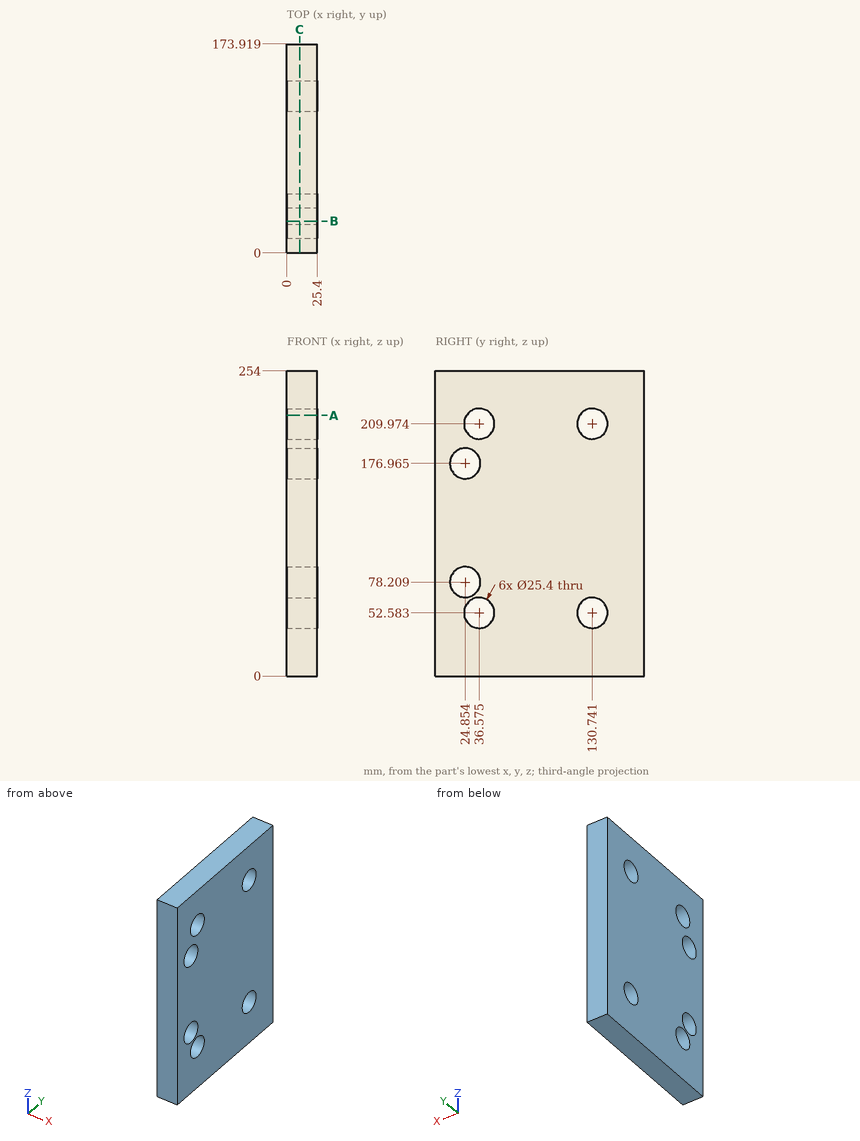
Drawing for the job (mm, zero at the part's lowest x, y, z). Round coordinates to 2 decimals unless told otherwise and drop trailing zeros. Write each loop counter-clockwise with the first axis right and the second up, starting at its lowest first coordinate (ties: lowest second). Pieces come first, ordered by that corner, then holes.
Item 1: Band-saw the part on B-B on y = 26.5. Give the number of separate pieces and of enclosed holes in the cut face, then the cut area to 3 significant figures.
Filled in:
separate pieces: 5
enclosed holes: 0
area: 4,390 mm2
Item 2: Band-saw the part on A-A on z = 217. Write the cut outline in (x, y) (1 decimal), then the cut area to 3 significant figures.
Filled in:
outline: (0, 0) - (25.4, 0) - (25.4, 26) - (0, 26) - close; (0, 47.2) - (25.4, 47.2) - (25.4, 120.2) - (0, 120.2) - close; (0, 141.3) - (25.4, 141.3) - (25.4, 173.9) - (0, 173.9) - close
area: 3,340 mm2
Item 3: Drill centre lines: L1, parallel to Y at x = 16.25, z = 177; L2, parallel to Y at x = 17.25, z = 221.5 (1 decimal); L3, parallel to Z at x = 14.5, y = 29 (1 decimal). Where is each one in solid material? Low to high.
Filled in:
L1: y = 0 to 12.15, 37.55 to 173.92
L2: y = 0 to 31.2, 41.9 to 125.4, 136.1 to 173.9
L3: z = 0 to 42.4, 62.8 to 66.2, 90.2 to 165, 189 to 199.8, 220.2 to 254
Item 4: Band-saw the part on C-C on x = 10.75. Write the cut outline in (y, z) (1 decimal), then the cut area to 3 significant figures.
Filled in:
outline: (0, 0) - (173.9, 0) - (173.9, 254) - (0, 254) - close; hole circle Ø25.4 at (24.9, 78.2); hole circle Ø25.4 at (24.9, 177); hole circle Ø25.4 at (36.6, 52.6); hole circle Ø25.4 at (36.6, 210); hole circle Ø25.4 at (130.7, 52.6); hole circle Ø25.4 at (130.7, 210)
area: 41,100 mm2
